Read the model definition and answer for the solid it produces. Units are mm, in the model's axes. A direction names the side the tool comes from. Round coordinates to 2 decimals unless told otherwise and drop trailing zeros. Loops run counter-clockwise (first coordinate to the right, second up) from the corner with the lowest first, then second, coordinate; pieces in that order, holes last. Notation, with made-up numbers: (72, 2) - (78, 2) arc R25 cw to (78, 36) - close; hole circle Ø10 at (-24.75, 10). An arc over 180 degrees is marked (long way). Answer as CSV lines item,"result".
Autodesk Inventor part; units mm, degrees
ref_plane "YZ Plane" through (0, 0, 0) normal (1, 0, 0) x (0, 1, 0)
ref_plane "XZ Plane" through (0, 0, 0) normal (0, 1, 0) x (-1, 0, 0)
ref_plane "XY Plane" through (0, 0, 0) normal (0, 0, 1) x (1, 0, 0)
sketch "Эскиз1" plane through (0, 0, 0) normal (0, 0, 1) x (1, 0, 0)
  line L0 (-54, -14) -> (54, -14)
  line L1 (54, -14) -> (54, 14)
  line L2 (54, 14) -> (-54, 14)
  line L3 (-54, 14) -> (-54, -14)
  line L4 (-54, -14) -> (54, 14) construction
  line L5 (54, -14) -> (-54, 14) construction
  point P0 (0, 0)
  dimension "d0" = 108
  dimension "d1" = 28
extrude "Выдавливание1" add sketch "Эскиз1" along normal blind 27.5
sketch "Эскиз2" plane through (0, 0, 27.5) normal (0, 0, 1) x (1, 0, 0)
  line L0 (-51, -11) -> (51, -11)
  line L1 (51, -11) -> (51, 11)
  line L2 (51, 11) -> (-51, 11)
  line L3 (-51, 11) -> (-51, -11)
  line L4 (-51, -11) -> (51, 11) construction
  line L5 (51, -11) -> (-51, 11) construction
  line L6 (54, 14) -> (-54, 14)
  line L7 (54, -14) -> (54, 14)
  point P0 (0, 0)
  dimension "d4" = 3
  dimension "d5" = 3
extrude "Выдавливание2" cut sketch "Эскиз2" against normal blind 24.5
sketch "Эскиз3" plane through (54, -14, 0) normal (1, 0, 0) x (0, 0, -1)
  line L0 (0, 28) -> (-27.5, 28)
  line L1 (0, 0) -> (-27.5, 0)
  line L2 (-27.5, 28) -> (-26, 28)
  line L3 (-26, 28) -> (-26, 0)
  line L4 (-26, 0) -> (-27.5, 0)
  line L5 (-27.5, 0) -> (-27.5, 28)
  point P0 (0, 14)
  dimension "d8" = 1.5
extrude "Выдавливание3" add sketch "Эскиз3" along normal blind 50
mirror "Зеркальное отражение1" about plane through (0, 0, 0) normal (1, 0, 0) of "Выдавливание3"
move faces "Перенос1" translate (6.5, 0, 0) faces at (104, 4.6667, 27)
move faces "Перенос2" translate (-6.5, 0, 0) faces at (-104, 4.6667, 27)
sketch "Эскиз7" plane through (-54, -14, 0) normal (0, -1, 0) x (1, 0, 0)
  line L0 (-56.5, 27.5) -> (164.5, 27.5)
  line L1 (0, 26) -> (-56.5, 26)
  line L2 (134, 27.5) -> (-26, 27.5)
  line L3 (-26, 27.5) -> (-26, 26)
  line L4 (-26, 26) -> (134, 26)
  line L5 (134, 26) -> (134, 27.5)
  line L6 (0, 0) -> (108, 0)
  point P0 (54, 0)
  point P1 (-26, 26.75)
  point P2 (54, 0)
  dimension "d29" = 160
  dimension "d30" = 80
extrude "Выдавливание7" add sketch "Эскиз7" along normal blind 2
sketch "Эскиз8" plane through (-54, 14, 0) normal (0, 1, 0) x (1, 0, 0)
  line L0 (-56.5, -27.5) -> (164.5, -27.5)
  line L1 (-26, -27.5) -> (134, -27.5)
  line L2 (134, -27.5) -> (134, 2)
  line L3 (134, 2) -> (-26, 2)
  line L4 (-26, 2) -> (-26, -27.5)
  line L5 (108, 0) -> (0, 0)
  point P0 (54, 0)
  point P1 (54, 0)
  dimension "d33" = 160
  dimension "d34" = 80
  dimension "d35" = 29.5
extrude "Выдавливание8" add sketch "Эскиз8" along normal blind 6
sketch "Эскиз9" plane through (80, 14, 26) normal (1, 0, 0) x (0, 0, -1)
  line L0 (28, 0) -> (28, 6)
  line L1 (28, 6) -> (-1.5, 6)
  line L2 (-1.5, 6) -> (-1.5, 2)
  line L3 (-1.5, 2) -> (28, 2)
  line L4 (28, 2) -> (28, 6)
  point P0 (26, -14)
  dimension "d38" = 4
extrude "Выдавливание9" add sketch "Эскиз9" along normal blind 29.5
mirror "Зеркальное отражение3" about plane through (0, 0, 0) normal (1, 0, 0) of "Выдавливание9"
sketch "Эскиз10" plane through (0, 0, 27.5) normal (0, 0, 1) x (1, 0, 0)
  circle A0 centre (-62.25, 0) radius 2
  circle A1 centre (62.25, 0) radius 2
  point P0 (0, 0)
extrude "Выдавливание10" cut sketch "Эскиз10" against normal through all
properties part number "000.009 - Короб" material "Пластик АБС"
1) The mould has two halves that part along Y. Classify faces 1 (the face through (60.252, 0.088, 26.76)), 2 (the face through (109.5, 18, 13)), 3 (the face through (2, 20, 13)): pulls with the +Y half, pulls with the -Y half, needs draft (parallel to the pull), parting line crosses it, or undercut.
Entries:
face 1,"undercut"
face 2,"needs draft"
face 3,"pulls with the +Y half"
2) Find the intervals of material crossed by line 1 (Y direction, x = -62.25, z = 26.3); line 2 (X direction, y = 2, z = 24.75); line 3 (Y direction, x = -7, z = 5.5), in increasing order.
Entries:
line 1,"y = -16 to -2, 2 to 20"
line 2,"x = -54 to -51, 51 to 54"
line 3,"y = -14 to -11, 11 to 20"
3) A cutting plane is placed at A-A, the plane y = 0. Determine the outline of the cut face in (x, z).
Entries:
outline,"(-110.5, 26) - (-64.25, 26) - (-64.25, 27.5) - (-110.5, 27.5) - close; (-60.25, 26) - (-54, 26) - (-54, 0) - (54, 0) - (54, 26) - (60.25, 26) - (60.25, 27.5) - (51, 27.5) - (51, 3) - (-51, 3) - (-51, 27.5) - (-60.25, 27.5) - close; (64.25, 26) - (110.5, 26) - (110.5, 27.5) - (64.25, 27.5) - close"
4) A cutting plane is placed at D-D, the plane x = -18. Determine the outline of the cut face in (y, z).
Entries:
outline,"(-16, 26) - (-14, 26) - (-14, 0) - (14, 0) - (14, -2) - (20, -2) - (20, 27.5) - (11, 27.5) - (11, 3) - (-11, 3) - (-11, 27.5) - (-16, 27.5) - close"
5) A cutting plane is placed at B-B, the plane x = 62.25. Determine the outline of the cut face in (y, z).
Entries:
outline,"(-16, 26) - (-2, 26) - (-2, 27.5) - (-16, 27.5) - close; (2, 26) - (14, 26) - (14, -2) - (20, -2) - (20, 27.5) - (2, 27.5) - close"
6) Each of these flat-tipped pins is pushed along its axis until it touches: P1, Ø6.5, axis at x = 62.25, y = 0, coming from the -Z side; P2, Ø6, axis at y = -7, z = 14, coming from the -X side; P3, Ø2, axis at x = 80, z = 16, coming from the -Y side. Where does it stop, or does it pass through?
Entries:
P1,"stops at z = 26"
P2,"stops at x = -54"
P3,"stops at y = 14"
7) A tool of negligible diameter and unlimited length cuts with its end or side. For faces 4 (the face through (-1, 0, 3)), 5 (the face through (1, -14, 13)), 6 (the face through (-60.403, -0.766, 26.76)), 7 (the face through (-54, 0, 13)), from which of +Z, -Z, +X, -X, +Y, -Y can it reach the whole face along a straight path? Write none if from no direction.
Entries:
face 4,"+Z"
face 5,"-Z, +X, -X, -Y"
face 6,"+Z, -Z"
face 7,"-Z, -X, -Y"
8) A cutting plane is placed at C-C, the plane z = 16. Determine the outline of the cut face in (x, y).
Entries:
outline,"(-109.5, 16) - (-80, 16) - (-80, 14) - (-54, 14) - (-54, -14) - (54, -14) - (54, 14) - (80, 14) - (80, 16) - (109.5, 16) - (109.5, 20) - (-109.5, 20) - close; hole (-51, -11) - (51, -11) - (51, 11) - (-51, 11) - close"
